Check sheet for the modelled part. Datum: model origin and axes. Units: mm. Round coordinates to 2 decimals unless told otherwise and drop trailing zeros. Order: outer loops, then holes, each group sorted by start corner. A loop starts at its lowest first (then second) coordinate and runs counter-clockwise, first axis right, second up.
```python
from build123d import *

# Parameters (mm, degrees)
SKETCH3_R                   = 3.81
DOWELSUPPORT_DEPTH          = 1.27
SKETCH5_W                   = 6.35
SKETCH5_H                   = 44.45
SLIDERDOWELSUPPORT_DEPTH    = 1.27
SKETCH17_R                  = 1.549999948
CUT_EXTRUDE1_DEPTH          = 19.685
CUT_EXTRUDE2_DEPTH          = 36.066505943
CUT_EXTRUDE2_DEPTH_BACK     = 36.066505943
SKETCH18_W                  = 1.27
SKETCH18_H                  = 25.4
LPATTERN1_COUNT             = 2
LPATTERN1_PITCH             = 25.4
LATERALSUPPORT_DEPTH        = 1.27
SKETCH8_W                   = 6.35
SKETCH8_H                   = 3
TABSUPPORT_DEPTH            = 1.27
STRINGDOWELSUPPORT_START    = -1.27
STRINGDOWELSUPPORT_DEPTH    = 5.08
INTERSUPPORT_DEPTH          = 1.27
SKETCH10_W                  = 6.35
SKETCH10_H                  = 3
TABBASE_DEPTH               = 1.27
SKETCH12_W                  = 6.35
SKETCH12_H                  = 3
TABDRAFT_DEPTH              = 1.73
TABDRAFT_DRAFT              = 5
TABDRAFT_PROFILE_2_DEPTH    = 1.73
TABDRAFT_PROFILE_2_DRAFT    = 5
STRINGDOWELHOLES_DEPTH      = 48.629791179
STRINGDOWELHOLES_DEPTH_BACK = 1.524
SKETCH14_R                  = 1.690500048
PULLEYDOWELHOLE_DEPTH       = 2.54
FILLET1_R                   = 6.35


with BuildPart() as part:
    # Sketch3 → DowelSupport (new, symmetric)
    with BuildSketch(Plane(origin=(0, 0, 0), x_dir=(0, 0, -1), z_dir=(1, 0, 0))):
        with Locations((0, 30.95625)):
            Circle(SKETCH3_R)
    extrude(amount=DOWELSUPPORT_DEPTH, both=True)

    # Sketch8 → TabSupport (add, symmetric)
    with BuildSketch(Plane(origin=(0, 0, 0), x_dir=(0, 0, -1), z_dir=(1, 0, 0))):
        with Locations((0, 27.94)):
            Rectangle(SKETCH8_W, SKETCH8_H)
        with Locations((-12.7, 27.94)):
            Rectangle(SKETCH8_W, SKETCH8_H)
    extrude(amount=TABSUPPORT_DEPTH, both=True)


with BuildPart() as body_2:
    # Sketch5 → SliderDowelSupport (new, symmetric)
    with BuildSketch(Plane(origin=(0, 0, 0), x_dir=(0, 0, -1), z_dir=(1, 0, 0))):
        Rectangle(SKETCH5_W, SKETCH5_H)
    extrude(amount=SLIDERDOWELSUPPORT_DEPTH, both=True)

    # Sketch17 → Cut-Extrude1 (cut, symmetric)
    with BuildSketch(Plane(origin=(0, 0, 0), x_dir=(1, 0, 0), z_dir=(0, 1, 0))):
        with Locations((0.482000052, 0)):
            Circle(SKETCH17_R)
        with BuildLine():
            Line((2.032, 0), (2.032, 1.399999994))
            Line((2.032, 1.399999994), (1.147206678, 1.399999994))
            ThreePointArc((1.147206678, 1.399999994), (1.792261491, 0.828078983), (2.032, 0))
        make_face()
        with BuildLine():
            Line((2.032, -1.399999994), (2.032, 0))
            ThreePointArc((2.032, 0), (1.792261491, -0.828078983), (1.147206678, -1.399999994))
            Line((1.147206678, -1.399999994), (2.032, -1.399999994))
        make_face()
    extrude(amount=CUT_EXTRUDE1_DEPTH, both=True, mode=Mode.SUBTRACT)

    # Sketch18 → Cut-Extrude2 (cut, two sides: drawn at the far end of the back side and taken through both)
    with BuildSketch(Plane.ZY.offset(1.27).offset(-CUT_EXTRUDE2_DEPTH_BACK)):
        Rectangle(SKETCH18_W, SKETCH18_H)
    extrude(amount=CUT_EXTRUDE2_DEPTH + CUT_EXTRUDE2_DEPTH_BACK, mode=Mode.SUBTRACT)


with BuildPart() as lpattern1_1:
    # LPattern1: pattern copy
    add(body_2.part.moved(Location(Vector(0, 0, 1) * (1 * LPATTERN1_PITCH))))


with BuildPart() as body_4:
    # Sketch6 → LateralSupport (new, symmetric)
    with BuildSketch(Plane(origin=(0, 0, 0), x_dir=(0, 0, -1), z_dir=(1, 0, 0))):
        Polygon((7.392863577, 33.391434671), (5.805363577, 36.141065329), (8.169612929, 37.506065329), (9.523465192, 37.701124423), (10.602965192, 35.831375577), (9.757112929, 34.756434671), align=None)
    extrude(amount=LATERALSUPPORT_DEPTH, both=True)


with BuildPart() as tabsupport_piece_1:
    # of the separate pieces the step leaves, piece 1, a body of its own (tabsupport_pieces)
    add(part.part.solids().sort_by_distance((1.27, 28.850193258, 3.175))[0])


with BuildPart() as tabsupport_piece_2:
    # of the separate pieces the step leaves, piece 2, a body of its own (tabsupport_pieces)
    add(part.part.solids().sort_by_distance((-1.27, 26.44, 9.525))[0])

    # Sketch15 → StringDowelSupport (add)
    with BuildSketch(Plane(origin=(0, 0, 0), x_dir=(0, 0, -1), z_dir=(1, 0, 0)).offset(STRINGDOWELSUPPORT_START)):
        with BuildLine():
            Line((-14.4145, 30.226), (-10.9855, 30.226))
            ThreePointArc((-10.9855, 30.226), (-8.6995, 27.94), (-10.9855, 25.654))
            Line((-10.9855, 25.654), (-14.4145, 25.654))
            ThreePointArc((-14.4145, 25.654), (-16.7005, 27.94), (-14.4145, 30.226))
        make_face()
    extrude(amount=STRINGDOWELSUPPORT_DEPTH)


with BuildPart() as body_2_1:
    add(body_2.part)

    add(lpattern1_1.part)  # InterSupport merges LPattern1_1

    add(body_4.part)  # InterSupport merges body 4

    add(tabsupport_piece_1.part)  # InterSupport merges TabSupport piece 1

    add(tabsupport_piece_2.part)  # InterSupport merges TabSupport piece 2
    # Sketch7 → InterSupport (add, symmetric)
    with BuildSketch(Plane(origin=(0, 0, 0), x_dir=(0, 0, -1), z_dir=(1, 0, 0))):
        Polygon((5.170363577, 37.240917591), (8.027863577, 32.291582409), (1.42875, 28.481582409), (-1.42875, 33.430917591), align=None)
        Polygon((-3.175, 15.875), (-3.175, 22.225), (3.175, 22.225), (3.175, 26.44), (0.923046602, 28.251940251), (-0.923046602, 33.660559749), (-10.9855, 30.226), (-14.4145, 30.226), (-15.109807039, 29.269115541), (-28.575, 22.225), (-22.225, 22.225), (-22.225, 0), (-3.175, 0), align=None)
    extrude(amount=INTERSUPPORT_DEPTH, both=True)

    # Sketch10 → TabBase (add)
    with BuildSketch(Plane.ZY.offset(1.27)):
        with Locations((0, 27.94)):
            Rectangle(SKETCH10_W, SKETCH10_H)
        with Locations((12.7, 27.94)):
            Rectangle(SKETCH10_W, SKETCH10_H)
    extrude(amount=TABBASE_DEPTH)


with BuildPart() as tabdraft_tool:
    # Sketch12 → TabDraft (with draft: the straight prism first)
    with BuildSketch(Plane.ZY.offset(2.54)):
        with Locations((0, 27.94)):
            Rectangle(SKETCH12_W, SKETCH12_H)
    extrude(amount=TABDRAFT_DEPTH)
    # TabDraft: the draft: its side faces are tilted about the plane it starts from
    tabdraft_sides = [tabdraft_tool.faces().sort_by_distance(p)[0] for p in [
        (-3.405, 27.94, 3.175),
        (-3.405, 29.44, 0),
        (-3.405, 27.94, -3.175),
        (-3.405, 26.44, 0),
    ]]
    draft(tabdraft_sides, Plane.ZY.offset(2.54), TABDRAFT_DRAFT)


with BuildPart() as body_2_2:
    add(body_2_1.part)

    # TabDraft: add tabdraft_tool
    add(tabdraft_tool.part)


with BuildPart() as tabdraft_profile_2_tool:
    # Sketch12 → TabDraft profile 2 (with draft: the straight prism first)
    with BuildSketch(Plane.ZY.offset(2.54)):
        with Locations((12.7, 27.94)):
            Rectangle(SKETCH12_W, SKETCH12_H)
    extrude(amount=TABDRAFT_PROFILE_2_DEPTH)
    # TabDraft profile 2: the draft: its side faces are tilted about the plane it starts from
    tabdraft_profile_2_sides = [tabdraft_profile_2_tool.faces().sort_by_distance(p)[0] for p in [
        (-3.405, 27.94, 9.525),
        (-3.405, 26.44, 12.7),
        (-3.405, 27.94, 15.875),
        (-3.405, 29.44, 12.7),
    ]]
    draft(tabdraft_profile_2_sides, Plane.ZY.offset(2.54), TABDRAFT_PROFILE_2_DRAFT)


with BuildPart() as body_2_3:
    add(body_2_2.part)

    # TabDraft profile 2: add tabdraft_profile_2_tool
    add(tabdraft_profile_2_tool.part)

    # Sketch16 → StringDowelHoles (cut, two sides: drawn at the far end of the back side and taken through both)
    with BuildSketch(Plane(origin=(1.27, 0, 0), x_dir=(0, 0, -1), z_dir=(1, 0, 0)).offset(-STRINGDOWELHOLES_DEPTH_BACK)):
        with BuildLine():
            Line((-12.905478326, 27.178), (-12.494521674, 27.178))
            ThreePointArc((-12.494521674, 27.178), (-9.294999952, 27.94), (-12.494521674, 28.702))
            Line((-12.494521674, 28.702), (-12.905478326, 28.702))
            ThreePointArc((-12.905478326, 28.702), (-16.105000048, 27.94), (-12.905478326, 27.178))
        make_face()
    extrude(amount=STRINGDOWELHOLES_DEPTH + STRINGDOWELHOLES_DEPTH_BACK, mode=Mode.SUBTRACT)

    # Sketch14 → PulleyDowelHole (cut)
    with BuildSketch(Plane(origin=(1.27, 0, 0), x_dir=(0, 0, -1), z_dir=(1, 0, 0))):
        with Locations((0, 30.95625)):
            Circle(SKETCH14_R)
    extrude(amount=-PULLEYDOWELHOLE_DEPTH, mode=Mode.SUBTRACT)

    # Mirror1: body 2 across plane


with BuildPart() as body_2_4:
    add(body_2_3.part)
    add(body_2_3.part.mirror(Plane.ZX))

    # Fillet1
    fillet1_edges = [body_2_4.edges().sort_by_distance(p)[0] for p in [
        (0, -22.225, 28.575),
        (0, 22.225, 28.575),
    ]]
    fillet(fillet1_edges, radius=FILLET1_R)


solid = body_2_4.part
```
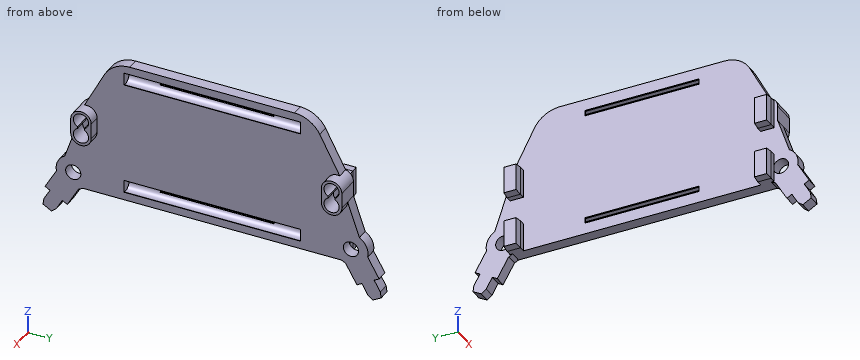
Item 1: Scan lines: line 1 along Z through (x, y) = (-1, -7.5) (3 decimals); line 2 along Y through (x, z) = (0.25, 1) (3 decimals); line 3 along Z through (x, y) = (1.3, 27.94) (1 decimal). Record each from-to range of solid material in increasing order.
Answer:
line 1: z = -3.175 to -0.635, 0.635 to 24.765, 26.035 to 28.575
line 2: y = -34.633 to -32.319, -29.593 to -19.685, 19.685 to 29.593, 32.319 to 34.633
line 3: z = 8.7 to 9.3, 16.1 to 16.7
Item 2: Sectioned sample at A-A (y = 7). Record the cut outline in (x, z) (3 decimals), and give its area (3 significant figures).
Answer:
outline: (-1.27, -3.175) - (1.27, -3.175) - (1.27, -1.4) - (1.147, -1.4) arc R1.55 cw to (-0.932, -0.635) - (-1.27, -0.635) - close; (-1.27, 0.635) - (-0.932, 0.635) arc R1.55 cw to (1.147, 1.4) - (1.27, 1.4) - (1.27, 24) - (1.147, 24) arc R1.55 cw to (-0.932, 24.765) - (-1.27, 24.765) - close; (-1.27, 26.035) - (-0.932, 26.035) arc R1.55 cw to (1.147, 26.8) - (1.27, 26.8) - (1.27, 28.575) - (-1.27, 28.575) - close
area: 67.8 mm2
Item 3: Go/stop test with flat-tipped pins: P1, Ø0.6, axis at x = -2, z = 12, coming from the -Y side; P2, Ø1.5, axis at x = 1, z = 8.5, coming from the -Y side; P3, Ø5, axis at y = 14, z = 0, coming from the +X side; P4, Ø1, axis at x = -2, y = -22, coming from the +Z side. Record where each tip stops, or that it passes through.
Answer:
P1: stops at y = -29.44
P2: stops at y = -31.33
P3: stops at x = 1.27
P4: passes through
Item 4: Sectioned sample at B-B (y = 21). Record the cut outline in (x, z) (3 decimals), and give its area (3 significant figures).
Answer:
outline: (-1.27, -3.175) - (1.27, -3.175) - (1.27, 28.01) - (-1.27, 28.01) - close
area: 79.2 mm2
